Drawing for the job (mm, zero at the part's lowest x, y, z). Give positions to 0.01 mm unless a question says otherwise; leave off trailing zeros. Order: outer loops, then holes, each group sorted by start corner. A loop starts at its lowest first (then second) coordinate and runs counter-clockwise, first axis right, second up. Notation, with made-up numbers: (-38.75, 88) - (-29.75, 88) arc R14 ccw to (-29.75, 112) - close; hole circle Ø1 at (-10.5, 81). An arc over 180 degrees is marked (long way). One line per item, written item: value.
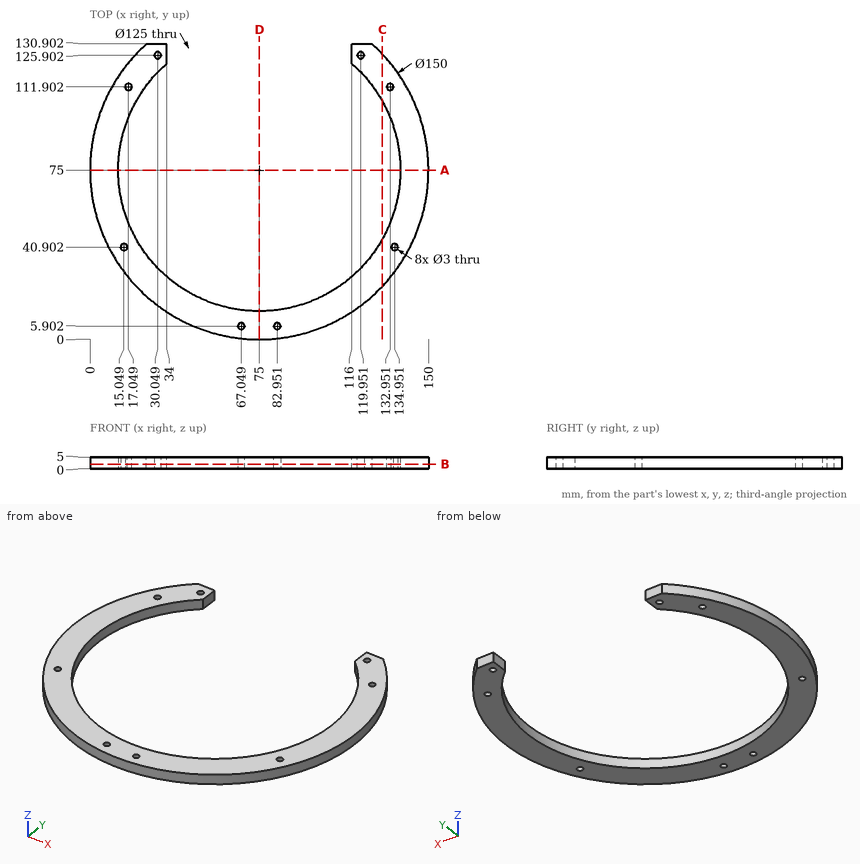
(1) Slice it at D-D, the plane x = 75. Give the cut face in (y, z), and give its area (3 significant figures).
Completed:
outline: (0, 0) - (12.5, 0) - (12.5, 5) - (0, 5) - close
area: 62.5 mm²
(2) Drill centre lines: line 1 (X direction, y = 75, z = 1.35); line 2 (Y direction, x = 29, z = 3.1) (1 decimal); line 3 (X direction, y = 84.5, z = 0.8). Where is each one in solid material? Low to high.
Completed:
line 1: 0 to 12.5, 137.5 to 150
line 2: 15.8 to 32.7, 117.3 to 124.8, 127 to 130.9
line 3: 0.6 to 13.23, 136.77 to 149.4
(3) Slice it at B-B, the plane z = 2. Count the separate pieces of the cut face and the enclosed holes in it, and give its area (3 significant figures).
Completed:
separate pieces: 1
enclosed holes: 8
area: 4,180 mm²
(4) Slice it at C-C, the plane x = 129.5. Give the cut face in (y, z), and give its area (3 significant figures).
Completed:
outline: (23.48, 0) - (44.41, 0) - (44.41, 5) - (23.48, 5) - close; (105.59, 0) - (126.52, 0) - (126.52, 5) - (105.59, 5) - close
area: 209 mm²
(5) Pin check, flat tips, straight feed: P1, Ø3.5, axis at x = 82.95, y = 5.9, coming from the -Z side; P2, Ø1.5, axis at y = 126.5, z = 3.5, coming from the -X side; P3, Ø2, axis at x = 113.5, z = 4.5, coming from the +Y side (1 decimal); P4, Ø3, axis at x = 36, z = 1.5, coming from the +Y side. Stop position of each tip, or through.
Completed:
P1: z = 0
P2: x = 19.78
P3: y = 26.6
P4: y = 27.4
(6) Slice it at A-A, the plane y = 75. Give the cut face in (x, z).
Completed:
outline: (0, 0) - (12.5, 0) - (12.5, 5) - (0, 5) - close; (137.5, 0) - (150, 0) - (150, 5) - (137.5, 5) - close
